```python
from build123d import *

# Parameters (mm, degrees)
F0_W     = 27.94
F0_H     = 20.32
F1_DEPTH = 12.7
F2_W     = 5.5372
F2_H     = 5.5372
F3_DEPTH = 18.542


# Not quite as in the source:
# - a feature names something its author has since deleted; it is built from what else it names


with BuildPart() as f1:
    # F0 (on Front) → F1 (new body)
    with BuildSketch(Plane.XZ):
        Rectangle(F0_W, F0_H)
    extrude(amount=F1_DEPTH)

    # F2 (on face) → F3 (cut)
    with BuildSketch(Plane.XY.offset(10.16)):
        with Locations((5.760986782, -6.0524168657)):
            Rectangle(F2_W, F2_H)
    extrude(amount=-F3_DEPTH, mode=Mode.SUBTRACT)


solid = f1.part
```
Could you check a few things on this model? Use its own coordinates, in mm. A direction names the side the tool comes from. Round coordinates to 2 decimals unless told otherwise and drop trailing zeros. Loops run counter-clockwise (first coordinate to the right, second up) from the corner with the lowest first, then second, coordinate; pieces in that order, holes last.
Q1. I want a section at A-A (z = -5). Write out the boundary of the cut face in (x, y), and give its area (3 significant figures).
Q2. On a 3-axis mill with a long thin cutter (end or side, diameter ignored), from which of +Z, -Z, +X, -X, +Y, -Y can I reach the whole of each face in a straight line? I mean faces 1 (the flat face through (0, 0, 0)), 2 (the flat face through (6, -6, -8.382)). Say none if no direction works.
Q3. I want a section at B-B (x = 6.75). Write out the boundary of the cut face in (y, z), and give its area (3 significant figures).
Q4. Please list where these lines run through material, in increasing order: L1, parallel to X at y = -7.5, z = -6.25; L2, parallel to Y at x = 4.75, z = 4; L3, parallel to Z at x = 7, y = -4.5.
Q5. I want a section at C-C (y = -6). Write out the boundary of the cut face in (x, z).
Q6. Thinking about a two-plate mould opening in X: for faces 3 (the flat face through (-13.97, -6, 0)), 4 (the flat face through (0, -6, 10.16)), 5 (the flat face through (6, -3.284, 1)), which applies, pulls with the +X half, pulls with the -X half, needs draft (parallel to the pull), parting line crosses it, or undercut?
Q7. For P1, Ø1.7, axis at x = 5, y = -6, coming from the +Z side, with a flat end and sliding along its axis, tell me the tip position at first contact or that it passes through.
Answer below:
1. outline: (-13.97, -12.7) - (13.97, -12.7) - (13.97, 0) - (-13.97, 0) - close; hole (2.99, -8.82) - (8.53, -8.82) - (8.53, -3.28) - (2.99, -3.28) - close
1. area: 324 mm2
2. face 1: +Z, -Z, +X, -X, +Y
2. face 2: +Z
3. outline: (-12.7, -10.16) - (0, -10.16) - (0, 10.16) - (-3.28, 10.16) - (-3.28, -8.38) - (-8.82, -8.38) - (-8.82, 10.16) - (-12.7, 10.16) - close
3. area: 155 mm2
4. L1: x = -13.97 to 2.99, 8.53 to 13.97
4. L2: y = -12.7 to -8.82, -3.28 to 0
4. L3: z = -10.16 to -8.38
5. outline: (-13.97, -10.16) - (13.97, -10.16) - (13.97, 10.16) - (8.53, 10.16) - (8.53, -8.38) - (2.99, -8.38) - (2.99, 10.16) - (-13.97, 10.16) - close
6. face 3: pulls with the -X half
6. face 4: needs draft
6. face 5: undercut
7. P1: stops at z = -8.38
